from build123d import *

# Parameters (mm, degrees)
SKETCH1_R           = 1.5
BOSS_EXTRUDE1_DEPTH = 6


with BuildPart() as part:
    # Sketch1 → Boss-Extrude1 (new body)
    with BuildSketch(Plane(origin=(0, 0, 0), x_dir=(0, 0, -1), z_dir=(1, 0, 0))):
        Polygon((0, 0), (0, 15), (103.223352982, 29.507096189), (101.831621972, 39.409776876), (66.916528588, 88.345571837), (71.800771975, 91.830419975), (107.568840624, 41.699124196), (110, 24.400526382), (22, 12.032932928), (22, 0), align=None)
        with Locations((4, 3)):
            Circle(SKETCH1_R, mode=Mode.SUBTRACT)
        with Locations((18, 3)):
            Circle(SKETCH1_R, mode=Mode.SUBTRACT)
    extrude(amount=BOSS_EXTRUDE1_DEPTH)


solid = part.part
Build history of the part. All positions in model axes, mm. A direction names the side the tool comes from. Round coordinates to 2 decimals unless told otherwise and drop trailing zeros. Loops run counter-clockwise (first coordinate to the right, second up) from the corner with the lowest first, then second, coordinate; pieces in that order, holes last. Notation, with made-up numbers: (26, 33) -> (48, 33) arc R24 ccw to (48, 55) -> close; hole circle Ø9 at (82, -0.5). An arc over 180 degrees is marked (long way). Answer in a Markdown table with one row per item.
Item 1: Which spindle directions (+Z, -Z, +X, -X, +Y, -Y) get a long thin tool onto all of the face, cutting with end or side? Do faces 1 (the flat face through (2.958, 34.389, -102.537)), 2 (the flat face through (0, 22, -59)), 3 (the flat face through (3, 6, -22)). Say none if no direction does.
Answers below:
| item | result |
|---|---|
| face 1 | +Z, +X, -X |
| face 2 | +Z, -Z, -X, +Y, -Y |
| face 3 | -Z, +X, -X, -Y |
Item 2: Saw through at C-C (x = 3.95). Write the cut outline in (y, z).
Answers below:
| item | result |
|---|---|
| outline | (0, -22) -> (12.03, -22) -> (24.4, -110) -> (41.7, -107.57) -> (91.83, -71.8) -> (88.35, -66.92) -> (39.41, -101.83) -> (29.51, -103.22) -> (15, 0) -> (0, 0) -> close; hole circle Ø3 at (3, -18); hole circle Ø3 at (3, -4) |
Item 3: Saw through at D-D (z = -4). Write the cut outline in (x, y).
Answers below:
| item | result |
|---|---|
| outline | (0, 0) -> (6, 0) -> (6, 1.5) -> (0, 1.5) -> close; (0, 4.5) -> (6, 4.5) -> (6, 15.56) -> (0, 15.56) -> close |
Item 4: Saw through at A-A (y = 3). Write the cut outline in (x, z), and give its area (3 significant figures).
Answers below:
| item | result |
|---|---|
| outline | (0, -22) -> (6, -22) -> (6, -19.5) -> (0, -19.5) -> close; (0, -16.5) -> (6, -16.5) -> (6, -5.5) -> (0, -5.5) -> close; (0, -2.5) -> (6, -2.5) -> (6, 0) -> (0, 0) -> close |
| area | 96.0 mm² |
Item 5: Drill centre lines: L1, parallel to Y at x = 2.6, z = -18; L2, parallel to Y at x = 0.35, z = -71; L3, parallel to Y at x = 4.3, z = -49. Where is each one in solid material? Low to high. Write a range as [from, to].
Answers below:
| item | result |
|---|---|
| L1 | y = [0, 1.5], [4.5, 17.53] |
| L2 | y = [18.92, 24.98], [82.62, 91.26] |
| L3 | y = [15.83, 21.89] |
Item 6: Pin check, flat tips, straight feed: pin 1 (2 mm diameter, centred on x = 1.5, z = -49, fed in from -Y); pin 2 (1 mm diameter, centred on x = 3, y = 39.5, fed in from -Z); pin 3 (3 mm diameter, centred on x = 2, z = -83, fed in from -Y). Stop position of each tip, or through.
Answers below:
| item | result |
|---|---|
| pin 1 | stops at y = 15.69 |
| pin 2 | stops at z = -107.95 |
| pin 3 | stops at y = 20.4 |
Item 7: Mould opens along Y. For faces 4 (the flat face through (3, 0, -11)), 5 (the flat face through (6, 22, -59)), 6 (the cylindrical face through (2.958, 2.425, -5.386)) say: +Y half, -Y half, draft (parallel to the pull), parting line (faces both ways), or undercut.
Answers below:
| item | result |
|---|---|
| face 4 | -Y half |
| face 5 | draft |
| face 6 | undercut |
Item 8: Saw through at B-B (z = -87.5). Write the cut outline in (x, y), and give its area (3 significant figures).
Answers below:
| item | result |
|---|---|
| outline | (0, 21.24) -> (6, 21.24) -> (6, 27.3) -> (0, 27.3) -> close; (0, 59.5) -> (6, 59.5) -> (6, 69.83) -> (0, 69.83) -> close |
| area | 98.3 mm² |
